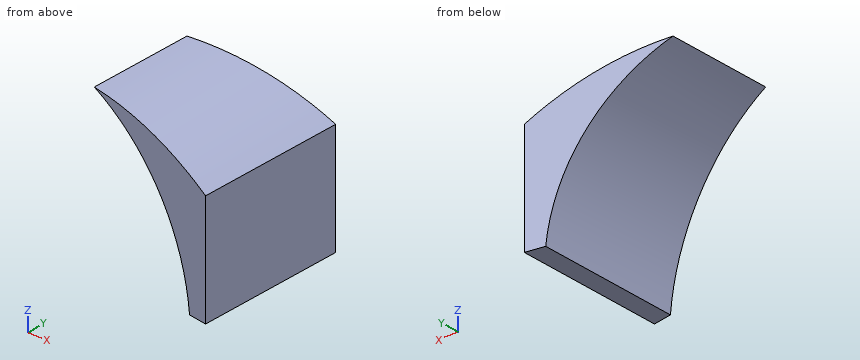
Autodesk Inventor part; units mm, degrees
ref_plane "YZ Plane" through (0, 0, 0) normal (1, 0, 0) x (0, 1, 0)
ref_plane "XZ Plane" through (0, 0, 0) normal (0, 1, 0) x (-1, 0, 0)
ref_plane "XY Plane" through (0, 0, 0) normal (0, 0, 1) x (1, 0, 0)
sketch "Sketch1" plane through (0, 0, 0) normal (0, 1, 0) x (-1, 0, 0)
  circle A0 centre (0, 0) radius 38.1
  line L0 (-38.1, 0) -> (-41.8338, 0)
  line L1 (-41.8338, 0) -> (-41.8338, 38.1)
  line L2 (-41.8338, 0) -> (-41.8338, -38.1)
  line L3 (-41.8338, -38.1) -> (0, -38.1)
  line L4 (0, 38.1) -> (-41.8338, 38.1)
  arc A1 (0, 38.1) -> (-38.1, 0) centre (0, 0) ccw
  arc A2 (0, 38.1) -> (-26.9408, 26.9408) centre (0, 0) ccw
  arc A3 (-38.1, 0) -> (0, -38.1) centre (0, 0) ccw
  arc A4 (-26.9408, -26.9408) -> (0, -38.1) centre (0, 0) ccw
  arc A5 (-14.5802, 35.1998) -> (-41.8338, 26.9408) centre (-12.1551, -21.8987) ccw
  arc A6 (-41.8338, -26.9408) -> (-14.5802, -35.1998) centre (-12.1551, 21.8987) ccw
  point P0 (-14.5802, -35.1998)
  dimension "d0" = 76.2
  dimension "d1" = 3.7338
  dimension "d2" = 57.15
  dimension "d3" = 57.15
extrude "Extrusion1" add sketch "Sketch1" against normal blind 31.75 contours A0 L0 L1 A5 | A6 L2 L0 A0
sketch "Sketch2" plane through (0, 0, 0) normal (0, 0, 1) x (1, 0, 0)
  line L0 (41.8338, -31.75) -> (-0.6683, -31.75)
  line L1 (41.8338, 0) -> (-9.3567, 0)
  line L2 (41.8338, 0) -> (-14.1234, -9.364)
  line L3 (41.8338, -31.75) -> (-10.3427, -23.0187)
  line L4 (7.8357, -38.2769) -> (6.8485, 14.5363)
  point P0 (0, 0)
  point P1 (7.1202, 0)
  point P2 (7.2285, -5.7909)
  point P3 (7.6066, -26.0223)
  point P4 (7.7137, -31.75)
  dimension "d6" = 9.5
  dimension "d7" = 9.5
extrude "Extrusion2" cut sketch "Sketch2" against normal mid plane 254
sketch "Sketch3" plane through (41.8338, 0, 26.9408) normal (-0.165, 0.9863, 0) x (0.9863, 0.165, 0)
  line L0 (-41.2601, 26.9408) -> (21.7895, 26.9408)
  line L1 (-41.2601, 30.7508) -> (21.7895, 30.7508)
  line L2 (-41.2601, 23.1308) -> (21.7895, 23.1308)
  line L3 (-30.0472, 14.0735) -> (-34.0912, 44.1278)
  line L4 (7.7274, 20.7829) -> (8.5546, 35.8559)
  line L5 (8.5546, 35.8559) -> (-7.3209, 76.3259)
  line L6 (-7.3209, 76.3259) -> (-43.5366, 68.5033)
  line L7 (-43.5366, 68.5033) -> (-33.4602, 39.4386)
  point P0 (7.8563, 23.1308)
  point P1 (-31.2659, 23.1308)
  dimension "d10" = 3.81
  dimension "d11" = 3.81
extrude "Extrusion3" cut sketch "Sketch3" against normal blind 254
sketch "Sketch4" plane through (0, 0, 0) normal (0, 1, 0) x (-1, 0, 0)
  line L0 (-41.8338, 3.81) -> (-37.909, 3.81)
  arc A0 (-14.5802, 35.1998) -> (-37.909, 3.81) centre (0, 0) ccw
  arc A1 (-14.5802, 35.1998) -> (-41.8338, 26.9408) centre (-12.1551, -21.8987) ccw
  line L1 (-41.8338, 26.9408) -> (-41.8338, 3.81)
  arc A2 (-14.5802, 35.1998) -> (-41.8338, 26.9408) centre (-12.1551, -21.8987) ccw
  line L2 (-14.5802, 35.1998) -> (-16.2152, 20.7478)
  dimension "d14" = 27.2536
  dimension "d15" = 31.3898
sketch "Sketch5" plane through (41.8338, -31.75, 26.9408) normal (1, 0, 0) x (0, 0, -1)
  line L0 (23.1308, 0) -> (0, 0)
  line L1 (0, 31.75) -> (23.1308, 31.75)
  point P0 (26.9408, 31.75)
  dimension "d16" = 31.75
properties part number "canister holder"
Part model, mm, in its own coordinate system. Round coordinates to 2 decimals unless told otherwise and drop trailing zeros. Write each loop counter-clockwise with the first axis right and the second up, starting at its lowest first coordinate (ties: lowest second). Pieces come first, ordered by that corner, then holes.
Item 1: Cut at B-B, the plane z = 17. Give the cut face in (x, y), plus the area to 3 significant figures.
Results:
outline: (34.1, -30.46) - (41.83, -31.75) - (41.83, 0) - (34.1, -1.29) - close
area: 236 mm2
Item 2: Cut at C-C, the plane y = -4. Give the cut face in (x, z).
Results:
outline: (17.93, 33.62) arc R38.1 cw to (37.91, 3.81) - (41.83, 3.81) - (41.83, 26.94) arc R57.15 ccw to (17.93, 34.96) - close
Item 3: Drop flat-ended pins along their axis: pin 1 Ø6 at (x, y) = (36, -16) entering from +Z; pin 2 Ø3 at (x, y) = (32, -10.5) entering from -Z; pin 3 Ø4 at (x, y) = (27, -17) entering from -Z. Give the stop position or say it passes through.
Results:
pin 1: stops at z = 31.31
pin 2: stops at z = 18.15
pin 3: stops at z = 24.71
Item 4: Cut at D-D, the plane y = -29.5. Give the cut face in (x, z), plus the area to 3 significant figures.
Results:
outline: (28.39, 25.41) arc R38.1 cw to (37.91, 3.81) - (41.83, 3.81) - (41.83, 26.94) arc R57.15 ccw to (28.39, 32.9) - close
area: 223 mm2
Item 5: Cut at A-A, the plane y = -15.5. Give the cut face in (x, z).
Results:
outline: (14.58, 35.2) arc R38.1 cw to (37.91, 3.81) - (41.83, 3.81) - (41.83, 26.94) arc R57.15 ccw to start
Item 6: Probe L1, parallel to Z at x = 34.5, y = -27.5; L2, parallel to Y at x = 37.75, z = 13; L3, parallel to Y at x = 39.5, z = 25.5. List the from-to ranges inside material, lowest first.
Results:
L1: z = 16.17 to 30.7
L2: y = -31.07 to -0.68
L3: y = -31.36 to -0.39
